Source: CAD feature listing. Evaluate the final solid. Frame: model axes, mm. Face numbers are marked on the shaded views. Give positions to 0.01 mm unless a question says otherwise; leave off trailing zeros. Write each loop counter-clockwise with the first axis right and the second up, starting at its lowest first coordinate (ties: lowest second). Pieces come first, ordered by that corner, then holes. Notation, with made-up numbers: (6, -5) -> (24, -5) arc R5 cw to (24, 4) -> close; hole circle Ø7 at (-32.75, 56). An arc over 180 degrees is marked (long way). Write item = value, one per line.
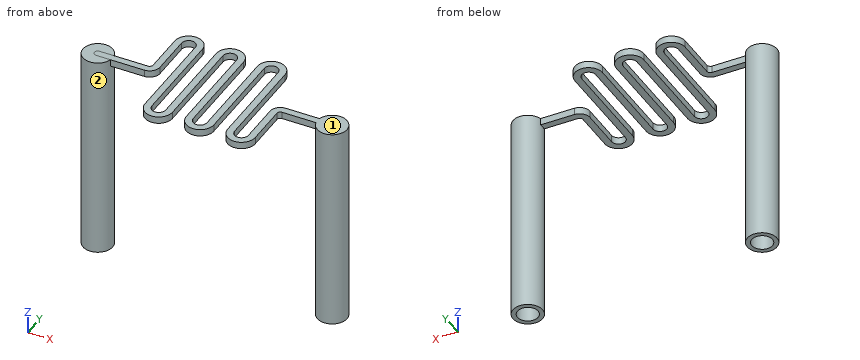
from build123d import *

# Parameters (mm, degrees)
BOSS_EXTRUDE1_DEPTH = 1
SKETCH3_W           = 2.15
SKETCH3_H           = 30
SKETCH4_W           = 2.15
SKETCH4_H           = 30
SKETCH5_R           = 1.5
CUT_EXTRUDE1_DEPTH  = 28
SKETCH6_R           = 1.5
CUT_EXTRUDE2_DEPTH  = 28


with BuildPart() as part:
    # Sketch2 → Boss-Extrude1 (new body)
    with BuildSketch(Plane.XY):
        with BuildLine():
            Line((-20.5, -0.5), (-13.5, -0.5))
            ThreePointArc((-13.5, -0.5), (-12.439339828, -0.060660172), (-12, 1))
            Line((-12, 1), (-12, 7))
            ThreePointArc((-12, 7), (-11, 8), (-10, 7))
            Line((-10, 7), (-10, 0))
            Line((-10, 0), (-10, -7))
            ThreePointArc((-10, -7), (-8, -9), (-6, -7))
            Line((-6, -7), (-6, 0))
            Line((-6, 0), (-6, 7))
            ThreePointArc((-6, 7), (-5, 8), (-4, 7))
            Line((-4, 7), (-4, 0))
            Line((-4, 0), (-4, -7))
            ThreePointArc((-4, -7), (-2, -9), (0, -7))
            Line((0, -7), (0, 0))
            Line((0, 0), (0, 7))
            ThreePointArc((0, 7), (1, 8), (2, 7))
            Line((2, 7), (2, 0))
            Line((2, 0), (2, -7))
            ThreePointArc((2, -7), (4, -9), (6, -7))
            Line((6, -7), (6, -1))
            ThreePointArc((6, -1), (6.146446609, -0.646446609), (6.5, -0.5))
            Line((6.5, -0.5), (13.5, -0.5))
            ThreePointArc((13.5, -0.5), (14, 0), (13.5, 0.5))
            Line((13.5, 0.5), (6.5, 0.5))
            ThreePointArc((6.5, 0.5), (5.439339828, 0.060660172), (5, -1))
            Line((5, -1), (5, -7))
            ThreePointArc((5, -7), (4, -8), (3, -7))
            Line((3, -7), (3, 0))
            Line((3, 0), (3, 7))
            ThreePointArc((3, 7), (1, 9), (-1, 7))
            Line((-1, 7), (-1, 0))
            Line((-1, 0), (-1, -7))
            ThreePointArc((-1, -7), (-2, -8), (-3, -7))
            Line((-3, -7), (-3, 0))
            Line((-3, 0), (-3, 7))
            ThreePointArc((-3, 7), (-5, 9), (-7, 7))
            Line((-7, 7), (-7, 0))
            Line((-7, 0), (-7, -7))
            ThreePointArc((-7, -7), (-8, -8), (-9, -7))
            Line((-9, -7), (-9, 0))
            Line((-9, 0), (-9, 7))
            ThreePointArc((-9, 7), (-11, 9), (-13, 7))
            Line((-13, 7), (-13, 1))
            ThreePointArc((-13, 1), (-13.146446609, 0.646446609), (-13.5, 0.5))
            Line((-13.5, 0.5), (-20.5, 0.5))
            ThreePointArc((-20.5, 0.5), (-21, 0), (-20.5, -0.5))
        make_face()
    extrude(amount=BOSS_EXTRUDE1_DEPTH)

    # Sketch3 → Revolve1 (revolve)
    with BuildSketch(Plane(origin=(0, 0, 0), x_dir=(1, 0, 0), z_dir=(0, 1, 0)), mode=Mode.PRIVATE) as revolve1_sk:
        with Locations((-21.575, 14.001632273)):
            Rectangle(SKETCH3_W, SKETCH3_H)
    revolve(revolve1_sk.sketch.rotate(Axis((-20.5, 0, 0.998367727), (0, 0, -1)), 180), axis=Axis((-20.5, 0, 0.998367727), (0, 0, -1)))

    # Sketch4 → Revolve2 (revolve)
    with BuildSketch(Plane(origin=(0, 0, 0), x_dir=(1, 0, 0), z_dir=(0, 1, 0))):
        with Locations((14.575, 14)):
            Rectangle(SKETCH4_W, SKETCH4_H)
    revolve(axis=Axis((13.5, 0, 1), (0, 0, -1)))

    # Sketch5 → Cut-Extrude1 (cut)
    with BuildSketch(Plane(origin=(0, 0, -29), x_dir=(-1, 0, 0), z_dir=(0, 0, -1))):
        with Locations((-13.5, 0)):
            Circle(SKETCH5_R)
        with Locations((20.5, 0)):
            Circle(SKETCH5_R)
    extrude(amount=-CUT_EXTRUDE1_DEPTH, mode=Mode.SUBTRACT)

    # Sketch6 → Cut-Extrude2 (cut)
    with BuildSketch(Plane(origin=(0, 0, -29.001632273), x_dir=(-1, 0, 0), z_dir=(0, 0, -1))):
        with Locations((20.5, 0)):
            Circle(SKETCH6_R)
    extrude(amount=-CUT_EXTRUDE2_DEPTH, mode=Mode.SUBTRACT)


solid = part.part
(1) First-contact query: pin 1 (2.5 mm diameter, centred on x = 13.5, y = 0, fed in from -Z); pin 2 (0.8 mm diameter, centred on x = 9, z = 0.5, fed in from +Y); pin 3 (1.1 mm diameter, centred on y = 2, z = 0.5, fed in from +X). Flat tips, straight axial feed; report the tip coordinate or a pass-through.
Values follow:
pin_1 = -1
pin_2 = 0.5
pin_3 = 15.09
(2) Section query A-A (y = 7.5). Return loops of the section in (x, z), plus the area to 3 significant figures.
Values follow:
outline = (-12.94, 0) -> (-11.87, 0) -> (-11.87, 1) -> (-12.94, 1) -> close; (-10.13, 0) -> (-9.06, 0) -> (-9.06, 1) -> (-10.13, 1) -> close; (-6.94, 0) -> (-5.87, 0) -> (-5.87, 1) -> (-6.94, 1) -> close; (-4.13, 0) -> (-3.06, 0) -> (-3.06, 1) -> (-4.13, 1) -> close; (-0.94, 0) -> (0.13, 0) -> (0.13, 1) -> (-0.94, 1) -> close; (1.87, 0) -> (2.94, 0) -> (2.94, 1) -> (1.87, 1) -> close
area = 6.42 mm2
(3) Section query B-B (x = 13.5). Return loops of the section in (y, z), plus the area to 3 significant figures.
Values follow:
outline = (-2.15, -29) -> (-1.5, -29) -> (-1.5, -1) -> (1.5, -1) -> (1.5, -29) -> (2.15, -29) -> (2.15, 1) -> (-2.15, 1) -> close
area = 45.0 mm2
(4) Section query C-C (z = -14). Return loops of the section in (x, y).
Values follow:
outline = circle Ø4.3 at (-20.5, 0); circle Ø4.3 at (13.5, 0); hole circle Ø3 at (-20.5, 0); hole circle Ø3 at (13.5, 0)
(5) Pull-direction query (X, two-part tool) for the marked faces 1 and 2; classes: pulls with the +X half, pulls with the -X half, needs draft (parallel to the pull), parting line crosses it, or undercut.
Values follow:
face_1 = needs draft
face_2 = undercut
(6) Section query D-D (y = 0). Give the number of separate pieces and of enclosed holes in the cut face, plus the area to 3 significant figures.
Values follow:
separate_pieces = 7
enclosed_holes = 0
area = 107 mm2
(7) Material intervals for line 1 (Y direction, x = -20.5, z = -19.5); line 2 (Z direction, x = -3.5, y = 6.75); line 3 (Y direction, x = 13, z = -15), sorted ascending.
Values follow:
line_1 = -2.15 to -1.5, 1.5 to 2.15
line_2 = 0 to 1
line_3 = -2.09 to -1.41, 1.41 to 2.09
